Autodesk Inventor part; units mm, degrees
ref_plane "Work Plane1" through (-9, 0, 0) normal (0, 0, 1) x (1, 0, 0)
ref_plane "Work Plane2" through (0, 0, -9) normal (-1, 0, 0) x (0, 0, 1)
ref_plane "YZ Plane" through (0, 0, 0) normal (1, 0, 0) x (0, 1, 0)
sketch "Sketch1" plane through (0, 0, 0) normal (0, 1, 0) x (-1, 0, 0)
  line L0 (-9, 9) -> (9, 9)
  line L1 (9, 9) -> (9, -9)
  line L2 (9, -9) -> (-9, -9)
  line L3 (-9, -9) -> (-9, 9)
  line L4 (-9, 9) -> (9, -9) construction
  line L5 (9, 9) -> (-9, -9) construction
  circle A0 centre (0, 0) radius 2
  line L6 (0, 0) -> (0, -6) construction
  circle A1 centre (0, -6) radius 2
  circle A2 centre (6, 0) radius 2
  circle A3 centre (0, 6) radius 2
  circle A4 centre (-6, 0) radius 2
  dimension "d0" = 18
  dimension "d1" = 18
  dimension "d2" = 4
  dimension "d3" = 6
  dimension "d8" = 4
  dimension "d11" = 360
extrude "Extrusion1" add sketch "Sketch1" along normal blind 3
sketch "Sketch2" plane through (0, 3, 0) normal (0, 1, 0) x (1, 0, 0)
  circle A0 centre (0, 6) radius 2
  circle A1 centre (0, 0) radius 2.5
  circle A2 centre (0, 6) radius 2.5
  circle A3 centre (-6, 0) radius 2.5
  circle A4 centre (0, -6) radius 2.5
  circle A5 centre (6, 0) radius 2.5
  dimension "d15" = 5
  dimension "d16" = 5
  dimension "d19" = 360
extrude "Extrusion2" cut sketch "Sketch2" against normal blind 0.8
sketch "Sketch3" plane through (0, 0, 0) normal (0, -1, 0) x (1, 0, 0)
  circle A0 centre (0, 0) radius 2.5
  circle A1 centre (0, -6) radius 2.5
  circle A2 centre (0, -6) radius 2.5
  circle A3 centre (6, 0) radius 2.5
  circle A4 centre (0, 6) radius 2.5
  circle A5 centre (-6, 0) radius 2.5
  dimension "d25" = 360
extrude "Extrusion3" cut sketch "Sketch3" against normal blind 0.8
sketch "Sketch4" plane through (9, 0, 9) normal (1, 0, 0) x (0, 0, -1)
  line L0 (0, 3) -> (3, 3) construction
  line L1 (0, 3) -> (18, 3)
  circle A0 centre (3, 3) radius 3
  point P0 (9, 0)
  dimension "d29" = 3
extrude "Extrusion4" add sketch "Sketch4" against normal blind 2.15
sketch "Sketch5" plane through (9, 0, 9) normal (1, 0, 0) x (0, 0, -1)
  line L0 (0, 3) -> (6, 3)
  arc A0 (6, 3) -> (0, 3) centre (3, 3) ccw
  circle A1 centre (3, 3) radius 2
  point P0 (9, 0)
  dimension "d32" = 4
extrude "Extrusion5" cut sketch "Sketch5" against normal blind 3 contours A1 L0 | L0 A1
sketch "Sketch6" plane through (9, 0, 9) normal (1, 0, 0) x (0, 0, -1)
  circle A0 centre (3, 3) radius 2
  circle A1 centre (3, 3) radius 2.5
  point P0 (9, 0)
  dimension "d35" = 5
extrude "Extrusion6" cut sketch "Sketch6" against normal blind 0.5
sketch "Sketch7" plane through (6.85, 0, 9) normal (-1, 0, 0) x (0, 0, 1)
  arc A0 (-1, 3) -> (-5, 3) centre (-3, 3) ccw
  circle A1 centre (-3, 3) radius 2.5
  point P0 (-9, 0)
  dimension "d38" = 5
extrude "Extrusion7" cut sketch "Sketch7" along normal blind 1
ref_plane "Work Plane1" through (-9, 0, 0) normal (0, 0, 1) x (1, 0, 0)
ref_plane "Work Plane2" through (0, 0, -9) normal (-1, 0, 0) x (0, 0, 1)
mirror "Mirror1" about plane through (-9, 0, 0) normal (0, 0, 1) of "Extrusion4", "Extrusion5", "Extrusion6", "Extrusion7"
mirror "Mirror2" about plane through (0, 0, -9) normal (-1, 0, 0) of "Extrusion4", "Extrusion5", "Extrusion6", "Extrusion7", "Mirror1"
properties part number "OlloHubToBase"
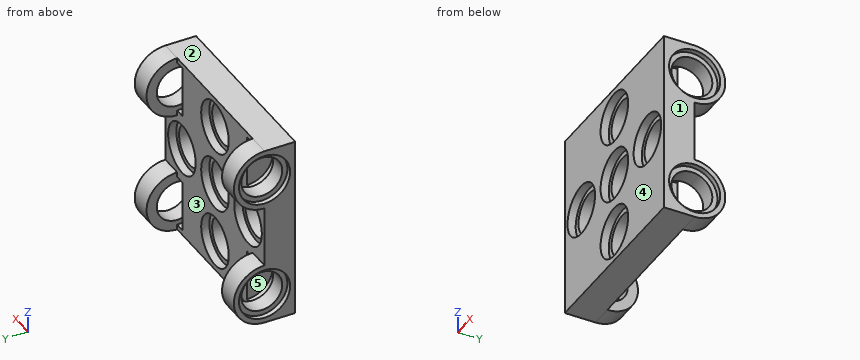
Work out the finished part from the listing and answer in its coordinate system (mm). Face numbers are marked on the shaded views. A direction names the side the tool comes from. Coordinates: 2 decimals unless noted, no trailing zeros. Write each loop counter-clockwise with the first axis right and the second up, starting at its lowest first coordinate (ties: lowest second). Pieces come first, ordered by that corner, then holes. Notation, with made-up numbers: M 50,61.25 L 103,61.25 A22 ccw 103,69.25 Z; hole C 48.5,15.5 d11. An arc over 180 degrees is marked long. Use one line per item in the form item = value. Start each with the question number.
1. The part is cut by section A-A (x = 5.5). Give the vertices of the cut face in (y, z).
2. Straight lines are drawn through the part: probe 1 along Z at (x, y) = (0, 1.2); probe 2 along Z at (x, y) = (0, 0.65); probe 3 along Y at (x, z) = (-8.75, 6). For each, find the intervals that lie inside material, in ascending order. Write a range as from..to.
3. A tool of negligible diameter and unlimited length cuts with its end or side. For the marked faces 4 and 5, from which of +Z, -Z, +X, -X, +Y, -Y can it reach the whole face along a straight path? Write none if from no direction.
4. Each of these flat-tipped pins is pushed along its axis until it touches: P1, Ø1, axis at y = 1.5, z = 6.5, coming from the +X side; P2, Ø5.5, axis at x = -3, z = 2.5, coming from the +Y side; P3, Ø2.5, axis at x = -6.5, z = 0, coming from the +Y side; P4, Ø5.5, axis at x = 6.5, z = 0.5, coming from the +Y side. Where does it stop, or does it pass through?
5. The mould has two halves that part along X. Classify the marked faces 1, 2 and 3: released by +X, released by -X, zero draft, split by the parting line, or undercut.
6. The part is cut by section B-B (z = -6). Give the number of separate pieces and of enclosed holes in the cut face, plus the area to 3 significant figures.
7. The part is cut by section D-D (z = 3.25). Give the vertices of the cut face in (x, y), plus the area to 3 significant figures.
Evaluation:
q1.outline = M 0,-9 L 3,-9 L 3,-2.45 L 2.2,-2.45 L 2.2,-1.94 L 0.8,-1.94 L 0.8,-2.45 L 0,-2.45 Z; M 0,2.45 L 0.8,2.45 L 0.8,1.94 L 2.2,1.94 L 2.2,2.45 L 3,2.45 L 3,9 L 0,9 Z
q2.probe_1 = -9..-8, -4..-2, 2..4, 8..9
q2.probe_2 = -9..-8.5, -3.5..-2.5, 2.5..3.5, 8.5..9
q2.probe_3 = 0..0.5, 5.5..6
q3.face_4 = +Z, -Z, +X, -X, -Y
q3.face_5 = +Y
q4.P1 = 8.5
q4.P2 = 3
q4.P3 = through
q4.P4 = 4.15
q5.face_1 = released by +X
q5.face_2 = zero draft
q5.face_3 = undercut
q6.separate_pieces = 4
q6.enclosed_holes = 0
q6.area = 30.1 mm^2
q7.outline = M -9,0 L 9,0 L 9,4.2 L 6.85,4.2 L 6.85,3 L -6.85,3 L -6.85,4.2 L -9,4.2 Z
q7.area = 59.2 mm^2
